Input: part model. Units: mm. Frame: model coordinates. A direction names the side the tool comes from. Round coordinates to 2 decimals unless told otherwise and drop trailing zeros. Loops run counter-clockwise (first coordinate to the right, second up) from the corner with the lowest first, then second, coordinate; pieces in that order, holes last. Notation, with made-up numbers: M 42,58.25 L 83,58.25 A7 cw 83,66.25 Z; hole C 51.25,-19.75 d3. An arc over 180 degrees is marked long. Use one line per item in the form item = value. Start each with the question number.
Q1. Section query C-C, the plane y = 19. Output: boundary loops of the cut face in (x, z), and give its area (3 significant figures).
Q2. Section query A-A, the plane z = 0. Output: boundary loops of the cut face in (x, y).
Q3. Access query for faces 5 (the flat face through (-3.5, 26, 0)), 6 (the flat face through (-2, 10, 2)). Directions: +Z, -Z, +X, -X, +Y, -Y. A direction counts if a zero-diameter tool reaches every point of the face in a straight line with its end or side. Return the directions, or none.
Q4. Section query B-B, the plane x = 0. Output: boundary loops of the cut face in (y, z).
Q5. Ray query, line 1 along X through (y, z) = (16, 0); line 2 along Y through (x, z) = (-1.25, 3.25). Return the intervals inside material, ascending.
Q6. Section query D-D, the plane y = 6.5. Output: boundary loops of the cut face in (x, z), and give its area (3 significant figures).
Q7. Mould query, pull axis X, two halves, no side actions, for faces 1 (the cylindrical face through (0, 27, 2)), 2 (the flat face through (0, 12, 0)), 3 (the flat face through (3.5, 26, 0)), 4 (the cylindrical face through (0, 5, 2)). Classes: pulls with the +X half, pulls with the -X half, needs draft (parallel to the pull), parting line crosses it, or undercut.
Q8. First-contact query: P1, Ø1.2, axis at x = -0.5, z = 0, coming from the +Y side; P2, Ø1, axis at y = 7.5, z = -2, coming from the -X side. Flat tips, straight axial feed; report the tip coordinate or a pass-through.
```python
from build123d import *

# Parameters (mm, degrees)
SKETCH1_R           = 2
BOSS_EXTRUDE1_DEPTH = 10
BOSS_EXTRUDE2_START = 10
SKETCH1_3_W         = 7
SKETCH1_3_H         = 7
BOSS_EXTRUDE2_DEPTH = 2
BOSS_EXTRUDE3_START = 12
SKETCH1_4_W         = 7
SKETCH1_4_H         = 7
SKETCH1_4_R         = 2
BOSS_EXTRUDE3_DEPTH = 30


with BuildPart() as part:
    # Sketch1 → Boss-Extrude1 (new body)
    with BuildSketch(Plane(origin=(0, 0, 0), x_dir=(1, 0, 0), z_dir=(0, 1, 0))):
        Circle(SKETCH1_R)
    extrude(amount=BOSS_EXTRUDE1_DEPTH)

    # Sketch1<3> → Boss-Extrude2 (add)
    with BuildSketch(Plane(origin=(0, 0, 0), x_dir=(1, 0, 0), z_dir=(0, 1, 0)).offset(BOSS_EXTRUDE2_START)):
        Rectangle(SKETCH1_3_W, SKETCH1_3_H)
    extrude(amount=BOSS_EXTRUDE2_DEPTH)

    # Sketch1<4> → Boss-Extrude3 (add)
    with BuildSketch(Plane(origin=(0, 0, 0), x_dir=(1, 0, 0), z_dir=(0, 1, 0)).offset(BOSS_EXTRUDE3_START)):
        Rectangle(SKETCH1_4_W, SKETCH1_4_H)
        Circle(SKETCH1_4_R, mode=Mode.SUBTRACT)
    extrude(amount=BOSS_EXTRUDE3_DEPTH)


solid = part.part
```
Results found:
q1.outline = M -3.5,-3.5 L 3.5,-3.5 L 3.5,3.5 L -3.5,3.5 Z; hole C 0,0 d4
q1.area = 36.4 mm²
q2.outline = M -3.5,10 L -2,10 L -2,0 L 2,0 L 2,10 L 3.5,10 L 3.5,42 L 2,42 L 2,12 L -2,12 L -2,42 L -3.5,42 Z
q3.face_5 = +Z, -Z, -X, +Y, -Y
q3.face_6 = -Y
q4.outline = M 0,-2 L 10,-2 L 10,-3.5 L 42,-3.5 L 42,-2 L 12,-2 L 12,2 L 42,2 L 42,3.5 L 10,3.5 L 10,2 L 0,2 Z
q5.line_1 = -3.5 to -2, 2 to 3.5
q5.line_2 = 10 to 42
q6.outline = C 0,0 d4
q6.area = 12.6 mm²
q7.face_1 = undercut
q7.face_2 = undercut
q7.face_3 = pulls with the +X half
q7.face_4 = parting line crosses it
q8.P1 = 12
q8.P2 = -1.32
